```python
from build123d import *

# Parameters (mm, degrees)
SKETCH_7_OUTSIDE_W  = 11.812
SKETCH_7_OUTSIDE_H  = 11.812
CUT_EXTRUDE_1_DEPTH = 2
CHAMFER_1_SIZE      = 0.3


with BuildPart() as part:
    # Эскиз1 → Повернуть1 (revolve)
    with BuildSketch(Plane.XY):
        Polygon((0, 0), (-2.25, 0), (-2.25, 3), (-3.7, 3), (-3.7, 6), (0, 6), align=None)
    revolve(axis=Axis((0, 0, 0), (0, 1, 0)))

    # Эскиз3 → Отверстие обработанное метчиком #6-321 (revolve, cut)
    with BuildSketch(Plane(origin=(0, 6, 0), x_dir=(0, 0, 1), z_dir=(1, 0, 0))):
        Polygon((0, 0), (0, 6), (1.8415, 6), (1.35255, 5.657633524), (1.35255, 0.342366476), (1.8415, 0), align=None)
    revolve(axis=Axis((0, 12.35, 0), (0, -1, 0)), mode=Mode.SUBTRACT)

    # Эскиз7 outside → Вырез-Вытянуть1 (cut)
    with BuildSketch(Plane(origin=(0, 6, 0), x_dir=(1, 0, 0), z_dir=(0, 1, 0))):
        Rectangle(SKETCH_7_OUTSIDE_W, SKETCH_7_OUTSIDE_H)
        Polygon((2.886751346, 0), (1.443375673, 2.5), (-1.443375673, 2.5), (-2.886751346, 0), (-1.443375673, -2.5), (1.443375673, -2.5), align=None, mode=Mode.SUBTRACT)
    extrude(amount=-CUT_EXTRUDE_1_DEPTH, mode=Mode.SUBTRACT)

    # Фаска1
    chamfer_1_edges = [part.edges().sort_by_distance(p)[0] for p in [
        (3.7, 4, 0),
    ]]
    chamfer(chamfer_1_edges, length=CHAMFER_1_SIZE)


solid = part.part
```
Work out the finished part from the listing and answer in its coordinate system (mm). A direction names the side the tool comes from. Give positions to 0.01 mm unless a question says otherwise; leave off trailing zeros. Order: outer loops, then holes, each group sorted by start corner. A loop starts at its lowest first (then second) coordinate and runs counter-clockwise, first axis right, second up. Notation, with made-up numbers: M 8,-33 L 41,-33 A17 ccw 41,-22 Z; hole C -36,-5 d9. An arc over 180 degrees is marked long. Return JSON: item names as keys, results as strings.
1) A tool of negligible diameter and unlimited length cuts with its end or side. For faces 5 (the flat face through (2.155, 5.014, 1.267)), 6 (the flat face through (0, 4, 3)), 7 (the cylindrical face through (0.29, 1.52, 2.23)), 8 (the flat face through (0, 5, -2.5)), from which of +Z, -Z, +X, -X, +Y, -Y can it reach the whole face along a straight path? Write none if from no direction.
Resolved:
{"face 5": "+Z, +X, +Y", "face 6": "+Y", "face 7": "-Y", "face 8": "-Z, +X, -X, +Y"}
2) This flat-tipped pin is pushed along its axis until it touches: pin 1 (1 mm diameter, centred on x = 0, y = 5.5, fed in from -Z). Where does it stop, or does it pass through?
Resolved:
{"pin 1": "z = -2.5"}
3) Section A-A, the plane x = 0 is taken. Write down the section's boundary in (y, z), plus the area to 3 significant figures.
Resolved:
{"outline": "M 0,-2.25 L 3,-2.25 L 3,-3.7 L 3.7,-3.7 L 4,-3.4 L 4,-2.5 L 6,-2.5 L 6,-1.84 L 5.66,-1.35 L 0.34,-1.35 L 0,-1.84 Z; M 0,1.84 L 0.34,1.35 L 5.66,1.35 L 6,1.84 L 6,2.5 L 4,2.5 L 4,3.4 L 3.7,3.7 L 3,3.7 L 3,2.25 L 0,2.25 Z", "area": "14.2 mm^2"}
4) Section B-B, the plane y = 4.8 is taken. Write down the section's boundary in (x, z).
Resolved:
{"outline": "M -2.89,0 L -1.44,-2.5 L 1.44,-2.5 L 2.89,0 L 1.44,2.5 L -1.44,2.5 Z; hole C 0,0 d2.71"}
5) Section C-C, the plane y = 0.9 is taken. Write down the section's boundary in (x, z), plus the area to 3 significant figures.
Resolved:
{"outline": "C 0,0 d4.5; hole C 0,0 d2.71", "area": "10.2 mm^2"}
6) For a pull along Z with two mould halves and no side action, classify faces 1 (the flat face through (0, 5, 2.5)), 2 (the flat face through (-2.155, 5.014, -1.267)), 3 (the cylindrical face through (-0.41, 3.04, 1.29)), 4 (the cylindrical face through (0.802, 3.355, -3.612)) as +Z half, -Z half, draft (parallel to the pull), parting line (faces both ways), or undercut.
Resolved:
{"face 1": "+Z half", "face 2": "-Z half", "face 3": "undercut", "face 4": "parting line"}
7) Straight lines are drawn through the part: line 1 along Z through (x, y) = (0, 2.6); line 2 along Y through (x, z) = (-0.75, -2.75); line 3 along Z through (x, y) = (0, 3.95). For each, find the intervals that lie inside material, in ascending order. Write a range as [from, to].
Resolved:
{"line 1": "[-2.25, -1.35], [1.35, 2.25]", "line 2": "[3, 4]", "line 3": "[-3.45, -1.35], [1.35, 3.45]"}
